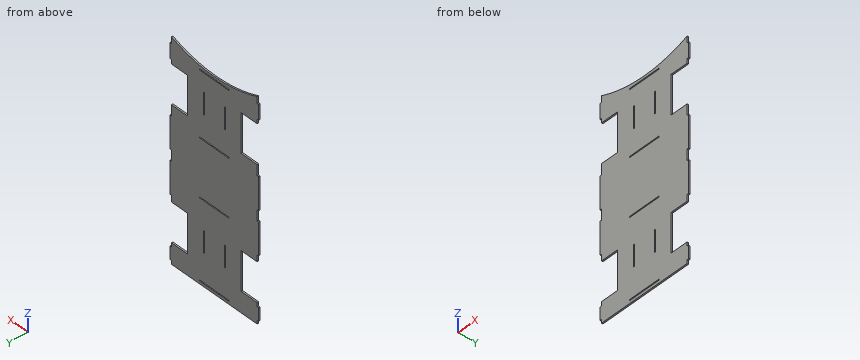
```python
from build123d import *

# Parameters (mm, degrees)
BOSS_EXTRUDE1_DEPTH = 1.3
SKETCH2_W           = 1.4
SKETCH2_H           = 12
SKETCH2_H_2         = 30
SKETCH2_H_3         = 14
BOSS_EXTRUDE2_DEPTH = 1.3
SKETCH3_W           = 30
SKETCH3_H           = 1
CUT_EXTRUDE1_DEPTH  = 110.421433001
SKETCH4_W           = 30
SKETCH4_H           = 1
CUT_EXTRUDE2_DEPTH  = 110.421433001
SKETCH6_W           = 30
SKETCH6_H           = 1
CUT_EXTRUDE3_DEPTH  = 110.421433001
SKETCH7_W           = 1
SKETCH7_H           = 20
SKETCH7_W_2         = 30
SKETCH7_H_2         = 1
CUT_EXTRUDE4_DEPTH  = 110.421433001
SKETCH8_W           = 1
SKETCH8_H           = 20
CUT_EXTRUDE5_DEPTH  = 110.421433001
SKETCH9_W           = 86
SKETCH9_H           = 1
BOSS_EXTRUDE3_DEPTH = 1.3


with BuildPart() as part:
    # Sketch1 → Boss-Extrude1 (new body)
    with BuildSketch(Plane(origin=(0, 0, 0), x_dir=(1, 0, 0), z_dir=(0, 1, 0))):
        with BuildLine():
            Line((43, 100), (-43, 100))
            Line((-43, 100), (-43, 82))
            Line((-43, 82), (-27, 82))
            Line((-27, 82), (-27, 46))
            Line((-27, 46), (-43, 46))
            Line((-43, 46), (-43, -40))
            Line((-43, -40), (-27, -40))
            Line((-27, -40), (-27, -76))
            Line((-27, -76), (-43, -76))
            Line((-43, -76), (-43, -100))
            ThreePointArc((-43, -100), (0, -91.240962318), (43, -100))
            Line((43, -100), (43, -76))
            Line((43, -76), (27, -76))
            Line((27, -76), (27, -40))
            Line((27, -40), (43, -40))
            Line((43, -40), (43, 46))
            Line((43, 46), (27, 46))
            Line((27, 46), (27, 82))
            Line((27, 82), (43, 82))
            Line((43, 82), (43, 100))
        make_face()
    extrude(amount=BOSS_EXTRUDE1_DEPTH)

    # Sketch2 → Boss-Extrude2 (add)
    with BuildSketch(Plane(origin=(0, 0, 0), x_dir=(1, 0, 0), z_dir=(0, 1, 0))):
        with Locations((43.7, 91.75)):
            Rectangle(SKETCH2_W, SKETCH2_H)
        with Locations((43.7, 25)):
            Rectangle(SKETCH2_W, SKETCH2_H_2)
        with Locations((43.7, -87)):
            Rectangle(SKETCH2_W, SKETCH2_H_3)
        with Locations((43.7, -15)):
            Rectangle(SKETCH2_W, SKETCH2_H_2)
    boss_extrude2 = extrude(amount=BOSS_EXTRUDE2_DEPTH)

    # Mirror1: Boss-Extrude2 across plane
    add(boss_extrude2.mirror(Plane(origin=(0, 0, 0), x_dir=(0, 0, 1), z_dir=(1, 0, 0))))

    # Sketch3 → Cut-Extrude1 (cut, through all)
    with BuildSketch(Plane(origin=(0, 1.3, 0), x_dir=(1, 0, 0), z_dir=(0, 1, 0))):
        with Locations((0, 98)):
            Rectangle(SKETCH3_W, SKETCH3_H)
    extrude(amount=-CUT_EXTRUDE1_DEPTH, mode=Mode.SUBTRACT)

    # Sketch4 → Cut-Extrude2 (cut, through all)
    with BuildSketch(Plane(origin=(0, 1.3, 0), x_dir=(1, 0, 0), z_dir=(0, 1, 0))):
        with Locations((0, -88.5)):
            Rectangle(SKETCH4_W, SKETCH4_H)
    extrude(amount=-CUT_EXTRUDE2_DEPTH, mode=Mode.SUBTRACT)

    # Sketch6 → Cut-Extrude3 (cut, through all)
    with BuildSketch(Plane(origin=(0, 1.3, 0), x_dir=(1, 0, 0), z_dir=(0, 1, 0))):
        with Locations((0, 24.5)):
            Rectangle(SKETCH6_W, SKETCH6_H)
    extrude(amount=-CUT_EXTRUDE3_DEPTH, mode=Mode.SUBTRACT)

    # Sketch7 → Cut-Extrude4 (cut, through all)
    with BuildSketch(Plane(origin=(0, 1.3, 0), x_dir=(1, 0, 0), z_dir=(0, 1, 0))):
        with Locations((-10.5, -61)):
            Rectangle(SKETCH7_W, SKETCH7_H)
        with Locations((10.5, -61)):
            Rectangle(SKETCH7_W, SKETCH7_H)
        with Locations((0, -28.5)):
            Rectangle(SKETCH7_W_2, SKETCH7_H_2)
    extrude(amount=-CUT_EXTRUDE4_DEPTH, mode=Mode.SUBTRACT)

    # Sketch8 → Cut-Extrude5 (cut, through all)
    with BuildSketch(Plane(origin=(0, 1.3, 0), x_dir=(1, 0, 0), z_dir=(0, 1, 0))):
        with Locations((-10.5, 61.25)):
            Rectangle(SKETCH8_W, SKETCH8_H)
        with Locations((10.5, 61.25)):
            Rectangle(SKETCH8_W, SKETCH8_H)
    extrude(amount=-CUT_EXTRUDE5_DEPTH, mode=Mode.SUBTRACT)

    # Sketch9 → Boss-Extrude3 (add)
    with BuildSketch(Plane(origin=(0, 0, 0), x_dir=(1, 0, 0), z_dir=(0, 1, 0))):
        with Locations((0, 100.5)):
            Rectangle(SKETCH9_W, SKETCH9_H)
    extrude(amount=BOSS_EXTRUDE3_DEPTH)


solid = part.part
```
Check sheet for the modelled part. Datum: model origin and axes. Units: mm. Round coordinates to 2 decimals unless told otherwise and drop trailing zeros. Order: outer loops, then holes, each group sorted by start corner. A loop starts at its lowest first (then second) coordinate and runs counter-clockwise, first axis right, second up. Notation, with made-up numbers: (25.25, -39) - (69.25, -39) arc R27 cw to (69.25, -15) - close; hole circle Ø8 at (-37, 39.5). An arc over 180 degrees is marked (long way). Answer as CSV lines item,"result". Start each with the question number.
1) Scan lines: probe 1 along X at (y, z) = (0.7, 70); probe 2 along Z at (x, y) = (0.5, 0.6); probe 3 along Z at (x, y) = (36.5, 0.7). Record each from-to range of solid material in increasing order.
2) Section check B-B (x = -8). Record the cut outline in (y, z).
3) Depth check by flat-ended pin: pin 1 (0.6 mm diameter, centred on x = -43.5, y = 0.5, fed in from -Z); pin 2 (0.6 mm diameter, centred on x = 39, y = 0.5, fed in from +Z); pin 3 (0.6 mm diameter, centred on x = -43.5, y = 0.5, fed in from +Z). Enter the tip coordinate at first touch or a pass-through.
4) Section check C-C (x = -38.5). Record the cut outline in (y, z), then the cut area to 3 significant figures.
5) Section check A-A (z = 57). Record the cut outline in (x, y).
6) Section check D-D (y = 0.7). Give the number of separate pieces and of enclosed holes in the cut face, then the cut area to 3 significant figures.
Determined:
1,probe 1,"-27 to -11, -10 to 10, 11 to 27"
1,probe 2,"-101 to -98.5, -97.5 to -25, -24 to 28, 29 to 88, 89 to 91.24"
1,probe 3,"-101 to -82, -46 to 40, 76 to 97.48"
2,outline,"(0, -101) - (1.3, -101) - (1.3, -98.5) - (0, -98.5) - close; (0, -97.5) - (1.3, -97.5) - (1.3, -25) - (0, -25) - close; (0, -24) - (1.3, -24) - (1.3, 28) - (0, 28) - close; (0, 29) - (1.3, 29) - (1.3, 88) - (0, 88) - close; (0, 89) - (1.3, 89) - (1.3, 91.53) - (0, 91.53) - close"
3,pin 1,"z = -97.75"
3,pin 2,"z = 98.51"
3,pin 3,"z = 94"
4,outline,"(0, -101) - (1.3, -101) - (1.3, -82) - (0, -82) - close; (0, -46) - (1.3, -46) - (1.3, 40) - (0, 40) - close; (0, 76) - (1.3, 76) - (1.3, 98.2) - (0, 98.2) - close"
4,area,"165 mm^2"
5,outline,"(-27, 0) - (-11, 0) - (-11, 1.3) - (-27, 1.3) - close; (-10, 0) - (10, 0) - (10, 1.3) - (-10, 1.3) - close; (11, 0) - (27, 0) - (27, 1.3) - (11, 1.3) - close"
6,separate pieces,"1"
6,enclosed holes,"8"
6,area,"14,500 mm^2"
